The listing builds one solid part. Answer for the finished solid, in the listing's coordinates (mm). A direction names the side the tool comes from. Coordinates: 2 decimals unless noted, no trailing zeros. Loops run counter-clockwise (first coordinate to the right, second up) from the corner with the lowest first, then second, coordinate; pieces in that order, holes last. Notation, with made-up numbers: (71, 15.25) - (108, 15.25) arc R29 ccw to (108, 44.25) - close; hole circle Ø6 at (74.25, -15). An arc over 180 degrees is marked (long way). Put each result on its own line as item: value.
```python
from build123d import *

# Parameters (mm, degrees)
SKETCH074_W             = 42.3
SKETCH074_H             = 42.3
PAD032_DEPTH            = 40
CHAMFER010_SIZE         = 3
SKETCH075_R             = 1.5
POCKET011_DEPTH         = 4.5
SKETCH076_R             = 11
PAD033_DEPTH            = 2
SKETCH077_R             = 2.5
PAD034_DEPTH            = 22
BODY017_ROLL_ANGLE      = 180
BODY017_PLACEMENT_ANGLE = 90


with BuildPart() as part:
    # Sketch074 → Pad032 (new body)
    with BuildSketch(Plane.XY):
        Rectangle(SKETCH074_W, SKETCH074_H)
    extrude(amount=PAD032_DEPTH)

    # Chamfer010
    chamfer010_edges = [part.edges().sort_by_distance(p)[0] for p in [
        (-21.15, -21.15, 20),
        (21.15, -21.15, 20),
        (21.15, 21.15, 20),
        (-21.15, 21.15, 20),
    ]]
    chamfer(chamfer010_edges, length=CHAMFER010_SIZE)

    # Sketch075 (on Face5 of Chamfer010) → Pocket011 (cut)
    with BuildSketch(Plane.XY.offset(40)):
        with Locations((15.5, -15.5)):
            Circle(SKETCH075_R)
        with Locations((-15.5, -15.5)):
            Circle(SKETCH075_R)
        with Locations((-15.5, 15.5)):
            Circle(SKETCH075_R)
        with Locations((15.5, 15.5)):
            Circle(SKETCH075_R)
    extrude(amount=-POCKET011_DEPTH, mode=Mode.SUBTRACT)

    # Sketch076 (on Face5 of Pocket011) → Pad033 (join)
    with BuildSketch(Plane.XY.offset(40)):
        Circle(SKETCH076_R)
    extrude(amount=PAD033_DEPTH)

    # Sketch077 (on Face19 of Pad033) → Pad034 (join)
    with BuildSketch(Plane.XY.offset(42)):
        Circle(SKETCH077_R)
    extrude(amount=PAD034_DEPTH)


with BuildPart() as part_1:
    # Body017 roll: moved
    add(part.part.rotate(Axis((0, 0, 0), (1, 0, 0)), BODY017_ROLL_ANGLE))


with BuildPart() as part_2:
    # Body017 placement: moved
    add(part_1.part.moved(Location((0, 67.5, -61))).rotate(Axis((0, 67.5, -61), (0, 0, 1)), BODY017_PLACEMENT_ANGLE))


solid = part_2.part
```
1) The part is cut by section C-C (y = 73). Give the vertices of the cut face in (x, z), and give its area (3 significant figures).
Found:
outline: (-21.15, -101) - (-9.53, -101) - (-9.53, -103) - (9.53, -103) - (9.53, -101) - (21.15, -101) - (21.15, -61) - (-21.15, -61) - close
area: 1,730 mm^2
2) Straight lines are drawn through the part: L1, parallel to X at y = 52, z = -98.95; L2, parallel to Z at x = -17, y = 85. For each, find the intervals that lie inside material, in ascending order. Write a range as [from, to].
Found:
L1: x = [-21.15, -17], [-14, 14], [17, 21.15]
L2: z = [-101, -61]
3) Each of these flat-tipped pins is pushed along its axis until it touches: pin 1 (2.5 mm diameter, centred on x = 16, y = 52, fed in from -Z); pin 2 (12 mm diameter, centred on y = 66.5, z = -116, fed in from +X); pin 3 (2.5 mm diameter, centred on x = -15.5, y = 52, fed in from -Z). Where does it stop, or does it pass through?
Found:
pin 1: stops at z = -101
pin 2: stops at x = 2.5
pin 3: stops at z = -96.5
4) For faces 4 (the face through (0.751, 69.885, -113.846)), 5 (the face through (-21.15, 67, -81)), determine the directions among +Z, -Z, +X, -X, +Y, -Y from which every point of the face is accessible in a straight line to the end or side of a thin tool.
Found:
face 4: -Z
face 5: +Z, -Z, -X, +Y, -Y
5) The part is cut by section B-B (x = 15.5). Give the vertices of the cut face in (y, z).
Found:
outline: (46.35, -101) - (50.5, -101) - (50.5, -96.5) - (53.5, -96.5) - (53.5, -101) - (81.5, -101) - (81.5, -96.5) - (84.5, -96.5) - (84.5, -101) - (88.65, -101) - (88.65, -61) - (46.35, -61) - close
6) For a pull along X with two mould halves and no side action, classify faces 1 (the face through (3, 67, -103)), 2 (the face through (-16.075, 84.386, -98.782)), 3 (the face through (-19.7, 47.9, -80.7)) as pulls with the +X half, pulls with the -X half, needs draft (parallel to the pull), parting line crosses it, or undercut.
Found:
face 1: needs draft
face 2: undercut
face 3: pulls with the -X half
7) The part is cut by section D-D (x = -13). Give the vertices of the cut face in (y, z), and give its area (3 significant figures).
Found:
outline: (46.35, -101) - (88.65, -101) - (88.65, -61) - (46.35, -61) - close
area: 1,690 mm^2
8) The part is cut by section A-A (y = 67.5). Give the vertices of the cut face in (x, z).
Found:
outline: (-21.15, -101) - (-11, -101) - (-11, -103) - (-2.5, -103) - (-2.5, -125) - (2.5, -125) - (2.5, -103) - (11, -103) - (11, -101) - (21.15, -101) - (21.15, -61) - (-21.15, -61) - close
